Source: CAD feature listing. Evaluate the final solid. Frame: model axes, mm. Face numbers are marked on the shaded views. Coordinates: 2 decimals unless noted, no trailing zeros. Loops run counter-clockwise (first coordinate to the right, second up) from the corner with the lowest first, then second, coordinate; pieces in that order, holes last.
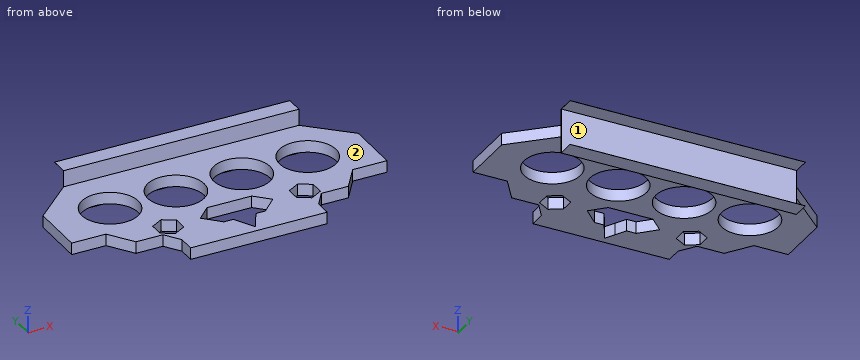
from build123d import *

# Parameters (mm, degrees)
SKETCH1_W           = 134
SKETCH1_H           = 63
BOSS_EXTRUDE1_DEPTH = 5
SKETCH3_R           = 12
CUT_EXTRUDE1_DEPTH  = 10
CUT_EXTRUDE2_DEPTH  = 10
BOSS_EXTRUDE2_DEPTH = 100


with BuildPart() as part:
    # Sketch1 → Boss-Extrude1 (new body)
    with BuildSketch(Plane.XY):
        Rectangle(SKETCH1_W, SKETCH1_H)
    extrude(amount=-BOSS_EXTRUDE1_DEPTH)

    # Sketch3 → Cut-Extrude1 (cut)
    with BuildSketch(Plane.XY):
        with Locations((-42, 9.071273883)):
            Circle(SKETCH3_R)
        with Locations((-14, 9.071273883)):
            Circle(SKETCH3_R)
        with Locations((14, 9.071273883)):
            Circle(SKETCH3_R)
        with Locations((42, 9.071273883)):
            Circle(SKETCH3_R)
    extrude(amount=-CUT_EXTRUDE1_DEPTH, mode=Mode.SUBTRACT)

    # Sketch4 → Cut-Extrude2 (cut)
    with BuildSketch(Plane.XY):
        Polygon((-67, -7.520628775), (-52.411804658, -7.520628775), (-45.12377265, -17.909951), (-33.648998849, -17.909951), (-29.023524966, -24.503711642), (-29.023524966, -31.5), (-67, -31.5), align=None)
        Polygon((67, -7.520628775), (67, -31.5), (29.023524966, -31.5), (29.023524966, -24.503711642), (33.648998849, -17.909951), (45.12377265, -17.909951), (52.411804658, -7.520628775), align=None)
        Polygon((-50, 31.5), (-67, 15.739047849), (-67, 31.5), align=None)
        Polygon((67, 15.739047849), (67, 31.5), (50, 31.5), align=None)
        Polygon((9.511401459, -7.520628775), (-9.511401459, -7.520628775), (-15.370004361, -13.379231677), (-8.815992906, -19.933243133), (-4.75570073, -19.933243133), (-2.290700849, -24.503711642), (0, -28.751004381), (2.290700849, -24.503711642), (4.75570073, -19.933243133), (8.815992906, -19.933243133), (15.370004361, -13.379231677), align=None)
        Polygon((-34.097223909, -10.449930226), (-29.023524966, -7.520628775), (-23.949826022, -10.449930226), (-23.949826022, -16.308533128), (-29.023524966, -19.237834579), (-34.097223909, -16.308533128), align=None)
        Polygon((29.023524966, -7.520628775), (23.949826022, -10.449930226), (23.949826022, -16.308533128), (29.023524966, -19.237834579), (34.097223909, -16.308533128), (34.097223909, -10.449930226), align=None)
    extrude(amount=-CUT_EXTRUDE2_DEPTH, mode=Mode.SUBTRACT)

    # Sketch5 → Boss-Extrude2 (add)
    with BuildSketch(Plane(origin=(50, 0, 0), x_dir=(0, 0, -1), z_dir=(1, 0, 0))):
        Polygon((5, 31.5), (12, 31.5), (12, 38.804238111), (11.980580676, 38.804238111), (11.980580676, 31.696116135), (5.980580676, 31.696116135), (-0.980580676, 31.696116135), (-6.980580676, 31.696116135), (-6.980580676, 38.804238111), (-7, 38.804238111), (-7, 31.5), (0, 31.5), align=None)
    extrude(amount=-BOSS_EXTRUDE2_DEPTH)


solid = part.part
Q1. Draft query along Y for the marked faces 1 and 2. Return one class per face: +Y half, -Y half, draft (parallel to the pull), parting line (faces both ways), or undercut.
Q2. Line query: line 1 along Y through (x, z) = (42, -2.75); line 2 along X through (y, z) = (5.5, -4.5); line 3 along Y through (x, z) = (-1.5, -1.75). Output: solid intervals per line, ascending.
Q3. Contact query for flat-ended pins moving along their axis: pin 1 Ø3 at (x, z) = (-41.5, -5) entering from -Y; pin 2 Ø2.5 at (y, z) = (-12.5, -3) entering from +X; pin 3 Ø6 at (x, y) = (-9, -1.5) entering from +Z. Output: stop coordinate, or through.
Q4. Section C-C, the plane x = -14. Count the separate pieces of the cut face and the enclosed holes in it, plus the area to 3 significant figures.
Q5. Section B-B, the plane y = 10.5. Return the cut outline in (x, z).
Derived:
1. face 1: +Y half
1. face 2: draft
2. line 1: y = -17.91 to -2.93, 21.07 to 31.7
2. line 2: x = -67 to -53.46, -30.54 to -25.46, -2.54 to 2.54, 25.46 to 30.54, 53.46 to 67
2. line 3: y = -31.5 to -25.97, -7.52 to 31.7
3. pin 1: stops at y = -17.91
3. pin 2: stops at x = 49.8
3. pin 3: stops at z = 0
4. separate pieces: 3
4. enclosed holes: 0
4. area: 185 mm2
5. outline: (-67, -5) - (-53.91, -5) - (-53.91, 0) - (-67, 0) - close; (-30.09, -5) - (-25.91, -5) - (-25.91, 0) - (-30.09, 0) - close; (-2.09, -5) - (2.09, -5) - (2.09, 0) - (-2.09, 0) - close; (25.91, -5) - (30.09, -5) - (30.09, 0) - (25.91, 0) - close; (53.91, -5) - (67, -5) - (67, 0) - (53.91, 0) - close
